from build123d import *

# Parameters (mm, degrees)
BOSS_EXTRUDE1_DEPTH     = 10
CUT_EXTRUDE1_DEPTH      = 67.219333
CUT_EXTRUDE2_DEPTH      = 2
M3_TAPPED_HOLE1_D       = 2.5
M3_TAPPED_HOLE1_DEPTH   = 9
M3_TAPPED_HOLE1_TIP     = 0.751076
SKETCH5_R               = 2.5
CUT_EXTRUDE3_DEPTH      = 44.185646
SKETCH6_R               = 4
CUT_EXTRUDE4_DEPTH      = 53.191953
CHAMFER1_SIZE           = 1
HOLE1_OUTLINE_R         = 2
HOLE1_DEPTH             = 30
HOLE1_START             = -16.200329
HOLE1_2_OUTLINE_R       = 1.25
HOLE1_2_DEPTH           = 16.200329
CUT_EXTRUDE5_REACH      = 54.192
CUT_EXTRUDE5_END_RADIUS = 7
SKETCH9_R               = 1.6
M4_TAPPED_HOLE1_REACH   = 68.219
M4_TAPPED_HOLE1_BORE_R  = 1.65
CUT_EXTRUDE6_REACH      = 68.219
CUT_EXTRUDE6_END_RADIUS = 2.5
SKETCH13_R              = 1.25


# Read off the part's stored shape, not the designer's step: Hole1
with BuildPart() as part:
    # Sketch1 → Boss-Extrude1 (new, symmetric)
    with BuildSketch(Plane.XY):
        Polygon((0, 0), (-19, 0), (-19, 32), (9, 32), (21, -6), (21, -30), (0, -30), align=None)
    extrude(amount=BOSS_EXTRUDE1_DEPTH, both=True)

    # Sketch2 → Cut-Extrude1 (cut, through all)
    with BuildSketch(Plane(origin=(0, 32, 0), x_dir=(1, 0, 0), z_dir=(0, 1, 0))):
        with BuildLine():
            ThreePointArc((-2.291796, 2), (-10.010587, 6.926667), (-16, 0))
            Line((-16, 0), (-2, 0))
            ThreePointArc((-2, 0), (-2.073333, 1.010587), (-2.291796, 2))
        make_face()
        with BuildLine():
            Line((-2, 0), (-16, 0))
            ThreePointArc((-16, 0), (-10.010587, -6.926667), (-2.291796, -2))
            ThreePointArc((-2.291796, -2), (-2.073333, -1.010587), (-2, 0))
        make_face()
    extrude(amount=-CUT_EXTRUDE1_DEPTH, mode=Mode.SUBTRACT)

    # Sketch2<3> → Cut-Extrude2 (cut)
    with BuildSketch(Plane(origin=(0, 32, 0), x_dir=(1, 0, 0), z_dir=(0, 1, 0))):
        with BuildLine():
            ThreePointArc((-2.291796, 2), (-2.073333, 1.010587), (-2, 0))
            Line((-2, 0), (3, 0))
            ThreePointArc((3, 0), (3.585786, 1.414214), (5, 2))
            Line((5, 2), (-2.291796, 2))
        make_face()
        with BuildLine():
            Line((3, 0), (-2, 0))
            ThreePointArc((-2, 0), (-2.073333, -1.010587), (-2.291796, -2))
            Line((-2.291796, -2), (5, -2))
            ThreePointArc((5, -2), (3.585786, -1.414214), (3, 0))
        make_face()
        with BuildLine():
            ThreePointArc((5, 2), (3.585786, 1.414214), (3, 0))
            Line((3, 0), (7, 0))
            ThreePointArc((7, 0), (6.414214, 1.414214), (5, 2))
        make_face()
        with BuildLine():
            Line((7, 0), (3, 0))
            ThreePointArc((3, 0), (3.585786, -1.414214), (5, -2))
            ThreePointArc((5, -2), (6.414214, -1.414214), (7, 0))
        make_face()
    extrude(amount=-CUT_EXTRUDE2_DEPTH, mode=Mode.SUBTRACT)

    # M3 Tapped Hole1
    with Locations(Plane(origin=(0, 32, 0), x_dir=(1, 0, 0), z_dir=(0, 1, 0))):
        with Locations((-16, 7), (-16, -7), (5, -7), (5, 7)):
            Hole(M3_TAPPED_HOLE1_D / 2, depth=M3_TAPPED_HOLE1_DEPTH)
            with Locations((0, 0, -(M3_TAPPED_HOLE1_DEPTH + M3_TAPPED_HOLE1_TIP / 2))):  # 118° drill point
                Cone(0, M3_TAPPED_HOLE1_D / 2, M3_TAPPED_HOLE1_TIP, mode=Mode.SUBTRACT)

    # Sketch5 → Cut-Extrude3 (cut, through all)
    with BuildSketch(Plane.XY.offset(10)):
        with Locations((13, -10)):
            Circle(SKETCH5_R)
    extrude(amount=-CUT_EXTRUDE3_DEPTH, mode=Mode.SUBTRACT)

    # Sketch6 → Cut-Extrude4 (cut, through all)
    with BuildSketch(Plane(origin=(21, 0, 0), x_dir=(0, 0, -1), z_dir=(1, 0, 0))):
        with Locations((0, -20)):
            Circle(SKETCH6_R)
    extrude(amount=-CUT_EXTRUDE4_DEPTH, mode=Mode.SUBTRACT)

    # Chamfer1
    chamfer1_edges = [part.edges().sort_by_distance(p)[0] for p in [
        (21, -20, 4),
    ]]
    chamfer(chamfer1_edges, length=CHAMFER1_SIZE)

    # Hole1 outline → Hole1 (cut)
    with BuildSketch(Plane(origin=(0, 0, 0), x_dir=(1, 0, 0), z_dir=(0, 1, 0))):
        with Locations((5, 0)):
            Circle(HOLE1_OUTLINE_R)
    extrude(amount=HOLE1_DEPTH, mode=Mode.SUBTRACT)

    # Hole1 2 outline → Hole1 2 (cut)
    with BuildSketch(Plane(origin=(0, 0, 0), x_dir=(1, 0, 0), z_dir=(0, 1, 0)).offset(HOLE1_START)):
        with Locations((5, 0)):
            Circle(HOLE1_2_OUTLINE_R)
    extrude(amount=HOLE1_2_DEPTH, mode=Mode.SUBTRACT)

    # Cut-Extrude5: up to this cylinder (the profile starts outside it)
    cut_extrude5_end = Plane(origin=(-9, 15, 0), z_dir=(0, 1, 0)) * Cylinder(CUT_EXTRUDE5_END_RADIUS, 123.384, mode=Mode.PRIVATE)
    # Sketch9 → Cut-Extrude5 (cut, up to the surface)
    with BuildSketch(Plane.ZY.offset(19), mode=Mode.PRIVATE) as cut_extrude5_sk1:
        with Locations(Location((-3, 15, 0), (0, 0, 270))):
            Circle(SKETCH9_R)
    cut_extrude5_tool1 = extrude(cut_extrude5_sk1.sketch, amount=-CUT_EXTRUDE5_REACH, mode=Mode.PRIVATE) - cut_extrude5_end
    add(cut_extrude5_tool1.solids().sort_by_distance((-19, 15, -3))[0], mode=Mode.SUBTRACT)
    # Sketch9 → Cut-Extrude5 (cut, up to the surface)
    with BuildSketch(Plane.ZY.offset(19), mode=Mode.PRIVATE) as cut_extrude5_sk2:
        with Locations(Location((3, 15, 0), (0, 0, 270))):
            Circle(SKETCH9_R)
    cut_extrude5_tool2 = extrude(cut_extrude5_sk2.sketch, amount=-CUT_EXTRUDE5_REACH, mode=Mode.PRIVATE) - cut_extrude5_end
    add(cut_extrude5_tool2.solids().sort_by_distance((-19, 15, 3))[0], mode=Mode.SUBTRACT)

    # M4 Tapped Hole1 bore → M4 Tapped Hole1 (cut, up to next)
    with BuildSketch(Plane(origin=(0, -30, 0), x_dir=(-1, 0, 0), z_dir=(0, -1, 0)), mode=Mode.PRIVATE) as m4_tapped_hole1_sk1:
        with Locations((-5, 0)):
            Circle(M4_TAPPED_HOLE1_BORE_R)
    m4_tapped_hole1_tool1 = extrude(m4_tapped_hole1_sk1.sketch, amount=-M4_TAPPED_HOLE1_REACH, mode=Mode.PRIVATE) & part.part
    # M4 Tapped Hole1 bore → M4 Tapped Hole1 (cut, up to next)
    with BuildSketch(Plane(origin=(0, -30, 0), x_dir=(-1, 0, 0), z_dir=(0, -1, 0)), mode=Mode.PRIVATE) as m4_tapped_hole1_sk2:
        with Locations((-13, 0)):
            Circle(M4_TAPPED_HOLE1_BORE_R)
    m4_tapped_hole1_tool2 = extrude(m4_tapped_hole1_sk2.sketch, amount=-M4_TAPPED_HOLE1_REACH, mode=Mode.PRIVATE) & part.part
    add(m4_tapped_hole1_tool1.solids().sort_by_distance((5, -30, 0))[0], mode=Mode.SUBTRACT)
    add(m4_tapped_hole1_tool2.solids().sort_by_distance((13, -30, 0))[0], mode=Mode.SUBTRACT)

    # Cut-Extrude6: up to this cylinder (the profile starts outside it)
    cut_extrude6_end = Plane(origin=(13, -10, 0), z_dir=(0, 0, 1)) * Cylinder(CUT_EXTRUDE6_END_RADIUS, 142.438, mode=Mode.PRIVATE)
    # Sketch13 → Cut-Extrude6 (cut, up to the surface)
    with BuildSketch(Plane.XZ.offset(30), mode=Mode.PRIVATE) as cut_extrude6_sk1:
        with Locations(Location((13, 0, 0), (0, 0, 270))):
            Circle(SKETCH13_R)
    cut_extrude6_tool1 = extrude(cut_extrude6_sk1.sketch, amount=-CUT_EXTRUDE6_REACH, mode=Mode.PRIVATE) - cut_extrude6_end
    add(cut_extrude6_tool1.solids().sort_by_distance((13, -30, 0))[0], mode=Mode.SUBTRACT)


solid = part.part
Read the model definition and answer for the solid it produces. Units are mm, in the model's axes. A direction names the side the tool comes from. Give positions to 0.01 mm unless a question says otherwise; leave off trailing zeros. Loops run counter-clockwise (first coordinate to the right, second up) from the corner with the lowest first, then second, coordinate; pieces in that order, holes last. Notation, with made-up numbers: (50.5, -11.5) -> (66.5, -11.5) arc R20 ccw to (66.5, 9.5) -> close; hole circle Ø4 at (-19.75, 45). An arc over 180 degrees is marked (long way). Use a Markdown table: item, result.
Q1. Section C-C, the plane y = -20 is taken. Determine the outline of the cut face in (x, z), then the cut area to 3 significant figures.
Solved:
| item | result |
|---|---|
| outline | (0, -10) -> (21, -10) -> (21, -5) -> (20, -4) -> (0, -4) -> close; (0, 4) -> (20, 4) -> (21, 5) -> (21, 10) -> (0, 10) -> close |
| area | 251 mm^2 |
Q2. A tool of negligible diameter and unlimited length cuts with its end or side. For faces 1 (the face through (-16, 0, 2)), 2 (the face through (-15.73, 27.44, -5.78)), 3 (the face through (-17.196, 15.208, 4.586)), from which of +Z, -Z, +X, -X, +Y, -Y can it reach the whole face along a straight path? Write none if from no direction.
Solved:
| item | result |
|---|---|
| face 1 | +Z, -Z, -X, -Y |
| face 2 | +Y |
| face 3 | -X |
Q3. Find the intervals of material crossed by line 1 along Z through (x, y) = (-17, 15); line 2 along Z through (x, y) = (5, 25); line 3 along Y through (x, z) = (8.5, 0), in increasing order.
Solved:
| item | result |
|---|---|
| line 1 | z = -10 to -4.6, -1.4 to 1.4, 4.6 to 10 |
| line 2 | z = -10 to -8.25, -5.75 to -2, 2 to 5.75, 8.25 to 10 |
| line 3 | y = -30 to -24, -16 to 32 |
Q4. Section A-A, the plane y = -10 is taken. Determine the outline of the cut face in (x, z).
Solved:
| item | result |
|---|---|
| outline | (0, -10) -> (10.5, -10) -> (10.5, 10) -> (0, 10) -> close; (15.5, -10) -> (21, -10) -> (21, 10) -> (15.5, 10) -> close; hole circle Ø2.5 at (5, 0) |
Q5. Section D-D, the plane x = -4.5 is taken. Determine the outline of the cut face in (y, z), then the cut area to 3 significant figures.
Solved:
| item | result |
|---|---|
| outline | (0, -10) -> (32, -10) -> (32, -5.36) -> (0, -5.36) -> close; (0, 5.36) -> (32, 5.36) -> (32, 10) -> (0, 10) -> close |
| area | 297 mm^2 |
Q6. Section B-B, the plane x = 1 is taken. Determine the outline of the cut face in (y, z), then the cut area to 3 significant figures.
Solved:
| item | result |
|---|---|
| outline | (-30, -10) -> (32, -10) -> (32, -2) -> (30, -2) -> (30, 2) -> (32, 2) -> (32, 10) -> (-30, 10) -> close; hole circle Ø8 at (-20, 0) |
| area | 1,180 mm^2 |
Q7. Determine the mould class of faces 4 (the face through (-15.73, 27.44, 8.22)), 5 (the face through (11, -30, 0)), 6 (the face through (1, 1, -10)) for opening direction Z: pulls with the +Z half, pulls with the -Z half, needs draft (parallel to the pull), parting line crosses it, or undercut.
Solved:
| item | result |
|---|---|
| face 4 | undercut |
| face 5 | needs draft |
| face 6 | pulls with the -Z half |
Q8. Each of these flat-tipped pins is pushed along its axis until it touches: pin 1 (6 mm diameter, centred on x = -2, z = -3, fed in from -Y); pin 2 (5 mm diameter, centred on y = -10.5, z = -2.5, fed in from -X); pin 3 (3 mm diameter, centred on x = 5, z = 0, fed in from +Y); pin 4 (5.5 mm diameter, centred on x = -7, z = -2, fed in from -Y). Where does it stop, or does it pass through?
Solved:
| item | result |
|---|---|
| pin 1 | stops at y = -30 |
| pin 2 | stops at x = 0 |
| pin 3 | stops at y = 0 |
| pin 4 | passes through |
